Geometry: final body of the model. Coordinates: model frame, mm. Face numbers are marked on the shaded views. A direction names the side the tool comes from. Coordinates: 2 decimals unless noted, no trailing zeros. Write each loop counter-clockwise with the first axis right and the second up, starting at its lowest first coordinate (ties: lowest second). Pieces come first, ordered by that corner, then holes. Notation, with made-up numbers: M 56.25,-12.75 L 77.25,-12.75 A12 ccw 77.25,10.25 Z; hole C -0.75,12 d2. An arc over 180 degrees is marked long. Write item = value, one per line. Start each with the question number.
Item 1: Ray query, L1, parallel to X at y = 14.5, z = 12; L2, parallel to X at y = -10, z = 19; L3, parallel to Z at x = 26, y = 3.5. Return the intervals inside material, ascending. Write a range as [from, to].
Item 2: Reachability of the marked faces 1, 2 and 3 from +Z, -Z, +X, -X, +Y, -Y: full face, straight path, thin tool, end or side. Return the list, or none.
Item 3: Section B-B on x = 85. Output: boundary loops of the cut face in (y, z).
Item 4: First-contact query: pin 1 Ø10 at (y, z) = (-15.5, 17.5) entering from +X; pin 2 Ø6 at (y, z) = (8.5, 18) entering from -X; pin 3 Ø5 at (x, y) = (30, 13) entering from +Z. Flat tips, straight axial feed; report the tip coordinate or a pass-through.
Item 5: Section A-A on x = 8.5. Output: boundary loops of the cut face in (y, z), plus the area to 3 significant figures.
Autodesk Inventor part; units mm, degrees
ref_plane "YZ Plane" through (0, 0, 0) normal (1, 0, 0) x (0, 1, 0)
ref_plane "XZ Plane" through (0, 0, 0) normal (0, 1, 0) x (-1, 0, 0)
ref_plane "XY Plane" through (0, 0, 0) normal (0, 0, 1) x (1, 0, 0)
sketch "スケッチ1" plane through (0, 0, 0) normal (0, 0, 1) x (1, 0, 0)
  line L0 (20.8, 7.5) -> (25, 7.5)
  line L1 (25, 7.5) -> (25, 21.05)
  line L2 (25, 21.05) -> (33, 21.05)
  line L3 (33, 21.05) -> (33, 23.15)
  line L4 (33, 23.15) -> (66.6, 23.15)
  line L5 (66.6, 23.15) -> (66.6, 21.05)
  line L6 (66.6, 21.05) -> (91.5, 21.05)
  line L7 (91.5, 21.05) -> (91.5, 7.5)
  line L8 (91.5, 7.5) -> (95.5, 7.5)
  line L9 (95.5, 7.5) -> (95.5, 2.5)
  line L10 (95.5, 2.5) -> (97, 2.5)
  line L11 (97, 2.5) -> (97, 0)
  line L12 (97, 0) -> (0, 0)
  line L13 (20.8, 7.5) -> (20.8, 2.5)
  line L14 (20.8, 2.5) -> (0, 2.5)
  line L15 (0, 2.5) -> (0, 0)
  dimension "d1" = 4.2
  dimension "d2" = 21.05
  dimension "d3" = 23.15
  dimension "d4" = 8
  dimension "d5" = 33.6
  dimension "d6" = 66.5
  dimension "d7" = 7.5
  dimension "d8" = 4
  dimension "d9" = 7.5
  dimension "d10" = 97
  dimension "d11" = 25
  dimension "d12" = 2.5
  dimension "d13" = 2.5
revolve "回転1" add sketch "スケッチ1" angle 360 about axis through (97, 0, 0) along (-1, 0, 0)
chamfer "面取り1" distance 1 angle 45 1 edges at (25, -21.05, 0)
fillet "フィレット1" radius 0.5 4 edges at (33, -23.15, 0) (66.6, -23.15, 0) (95.5, -7.5, 0) (97, -2.5, 0)
properties part number "RS-775"
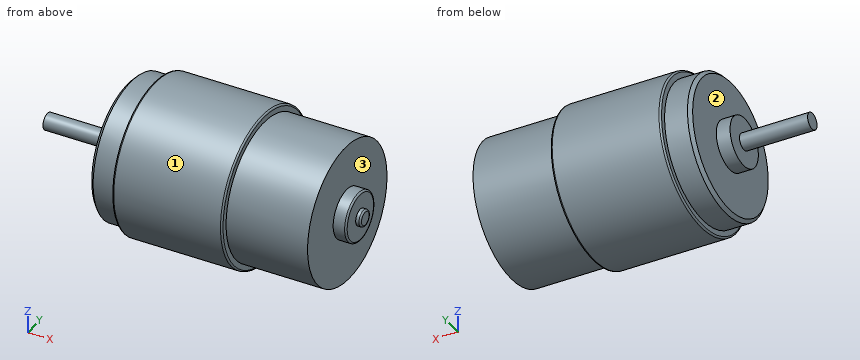
Responses:
q1.L1 = [25, 91.5]
q1.L2 = [33, 66.6]
q1.L3 = [-20.76, 20.76]
q2.face_1 = +X, -X
q2.face_2 = -X
q2.face_3 = +X
q3.outline = C 0,0 d42.1
q4.pin_1 = 91.5
q4.pin_2 = 25
q4.pin_3 = 18.24
q5.outline = C 0,0 d5
q5.area = 19.6 mm²
